from build123d import *

# Parameters (mm, degrees)
REDONDEO1_R           = 1
CHAFL_N1_SIZE         = 1
CORTAR_EXTRUIR1_START = -12.000013
CROQUIS2_R            = 18.122324433
CORTAR_EXTRUIR1_DEPTH = 12.000014
REDONDEO3_R           = 0.5


with BuildPart() as part:
    # Croquis1 → Revolución1 (revolve)
    with BuildSketch(Plane.XY, mode=Mode.PRIVATE) as revoluci_n1_sk:
        with BuildLine():
            Line((0, 0), (0, 17.3))
            Line((0, 17.3), (12, 17.3))
            Line((12, 17.3), (12, 10))
            Line((12, 10), (46, 10))
            ThreePointArc((46, 10), (46.5, 9.5), (47, 10))
            Line((47, 10), (72, 10))
            Line((72, 10), (72, 0))
            Line((72, 0), (0, 0))
        make_face()
    revolve(revoluci_n1_sk.sketch.rotate(Axis((72, 0, 0), (-1, 0, 0)), 90), axis=Axis((72, 0, 0), (-1, 0, 0)))

    # Redondeo1
    redondeo1_edges = [part.edges().sort_by_distance(p)[0] for p in [
        (12, 0, 17.3),
        (12, 0, 10),
    ]]
    fillet(redondeo1_edges, radius=REDONDEO1_R)

    # Chaflán1
    chafl_n1_edges = [part.edges().sort_by_distance(p)[0] for p in [
        (72, 0, 10),
    ]]
    chamfer(chafl_n1_edges, length=CHAFL_N1_SIZE)

    # Croquis4 → Cortar-Revolución1 (revolve, cut)
    with BuildSketch(Plane.XY, mode=Mode.PRIVATE) as cortar_revoluci_n1_sk:
        Polygon((0, 17.3), (0, 15.3), (2, 17.3), align=None)
    revolve(cortar_revoluci_n1_sk.sketch.rotate(Axis((0, 0, 0), (1, 0, 0)), 270), axis=Axis((0, 0, 0), (1, 0, 0)), mode=Mode.SUBTRACT)

    # Croquis2 → Cortar-Extruir1 (cut)
    with BuildSketch(Plane.ZY.offset(CORTAR_EXTRUIR1_START)):
        Circle(CROQUIS2_R)
        Polygon((8.65, 14.982239485), (-8.65, 14.982239485), (-17.3, 0), (-8.65, -14.982239485), (8.65, -14.982239485), (17.3, 0), align=None, mode=Mode.SUBTRACT)
    extrude(amount=CORTAR_EXTRUIR1_DEPTH, mode=Mode.SUBTRACT)

    # Redondeo3
    redondeo3_edges = [part.edges().sort_by_distance(p)[0] for p in [
        (6.5, 14.982239485, 8.65),
        (6.5, 0, 17.3),
        (6.5, -14.982239485, 8.65),
        (6.5, 14.982239485, -8.65),
        (6.5, 0, -17.3),
        (6.5, -14.982239485, -8.65),
    ]]
    fillet(redondeo3_edges, radius=REDONDEO3_R)


solid = part.part
Check sheet for the modelled part. Datum: model origin and axes. Units: mm. A direction names the side the tool comes from. Give positions to 0.01 mm unless a question says otherwise; leave off trailing zeros. Loops run counter-clockwise (first coordinate to the right, second up) from the corner with the lowest first, then second, coordinate; pieces in that order, holes last. Notation, with made-up numbers: M 55.25,41.25 L 87.25,41.25 A30 cw 87.25,78.25 Z; hole C 23,68.25 d5. An arc over 180 degrees is marked long. Answer as a JSON object with one key per item and string values. Group by question number.
Q1. Go/stop test with flat-tipped pins: P1, Ø1, axis at x = 43.5, z = 4.5, coming from the -Y side; P2, Ø4, axis at x = 49, z = 12.5, coming from the +Y side; P3, Ø5, axis at x = 29, y = -1, coming from the +Z side; P4, Ø6, axis at x = 8.5, y = -8.5, coming from the +Z side. Record where each tip stops, or that it passes through.
Q2. Cross-section at C-C on x = 24. Record the cut outline in (y, z), then the cut area to 3 significant figures.
Q3. Access from +Z, -Z, +X, -X, +Y, -Y to the whole of each face (thin tool, end or side, straight path). Record for faces 1 (the conical face through (0.548, 13.76, 7.862)), 2 (the cylindrical face through (59, 0, 10)).
Q4. Material ranges on line 1 along X through (y, z) = (-10.25, -7.5); line 2 along Z through (x, y) = (25, -0.5); line 3 along Y through (x, z) = (36.5, 5.5), recorded low to high. Write a range as [from, to].
Q5. Cross-section at B-B on x = 6. Record the cut outline in (y, z), then the cut area to 3 significant figures.
Q6. Cross-section at A-A on z = 0. Record the cut outline in (x, y), then the cut area to 3 significant figures.
Evaluation:
{
 "1": {"P1": "stops at y = -9.17", "P2": "passes through", "P3": "stops at z = 10", "P4": "stops at z = 14.12"},
 "2": {"outline": "C 0,0 d20", "area": "314 mm2"},
 "3": {"face 1": "+Z, -X, +Y", "face 2": "+X"},
 "4": {"line 1": "x = [0, 12]", "line 2": "z = [-9.99, 9.99]", "line 3": "y = [-8.35, 8.35]"},
 "5": {"outline": "M -14.98,-8.36 A0.5 ccw -14.73,-8.79 L -0.25,-17.16 A0.5 ccw 0.25,-17.16 L 14.73,-8.79 A0.5 ccw 14.98,-8.36 L 14.98,8.36 A0.5 ccw 14.73,8.79 L 0.25,17.16 A0.5 ccw -0.25,17.16 L -14.73,8.79 A0.5 ccw -14.98,8.36 Z", "area": "777 mm2"},
 "6": {"outline": "M 0,-14.98 L 12,-14.98 L 12,-11 A1 cw 13,-10 L 46,-10 A0.5 cw 47,-10 L 71,-10 L 72,-9 L 72,9 L 71,10 L 47,10 A0.5 cw 46,10 L 13,10 A1 cw 12,11 L 12,14.98 L 0,14.98 Z", "area": "1,560 mm2"}
}
